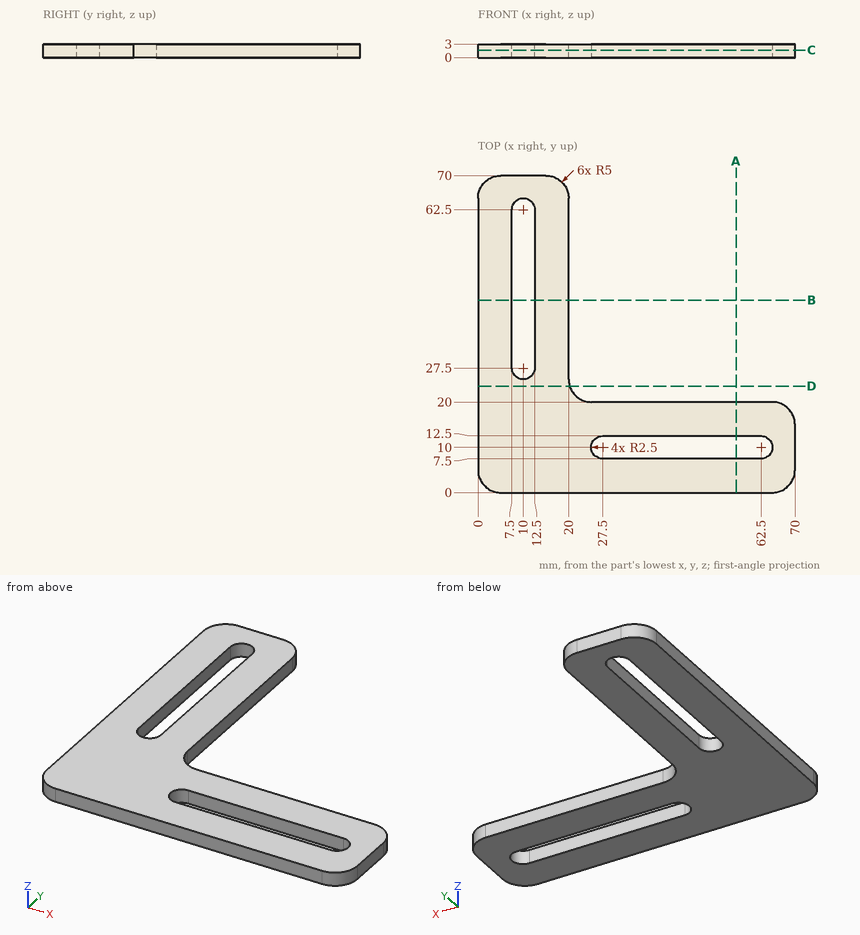
Source: three-view drawing plus pictorial views. Frame: mm from the lowest corner of the part. Coordinates: 2 decimals unless noted, no trailing zeros. Loops run counter-clockwise (first coordinate to the right, second up) from the corner with the lowest first, then second, coordinate; pieces in that order, holes last. Notation, with made-up numbers: (-39.5, 15.5) - (15.5, 15.5) arc R10 ccw to (15.5, 28.5) - close; hole circle Ø1 at (-34.5, 44). An arc over 180 degrees is marked (long way). Answer in a Markdown table with one row per item. Add a question column.
Item 1: Contact query for flat-ended pins moving along their axis: P1, Ø0.9, axis at y = 43.5, z = 2, coming from the +X side; P2, Ø1.5, axis at x = 49.5, z = 1, coming from the +Y side. Output: stop coordinate, or through.
Item 2: Section query A-A on x = 57. Return the cut outline in (y, z).
Item 3: Section query D-D on y = 23.5. Return the cut outline in (x, z).
Item 4: Section query C-C on z = 1.65. Return the cut outline in (x, y).
Item 5: Line query: line 1 along Y through (x, z) = (53, 2.4); line 2 along Y through (x, z) = (10, 1.1). Output: solid intervals per line, ascending. Write a range as [from, to].
Recorded:
| question | item | result |
|---|---|---|
| 1 | P1 | x = 20 |
| 1 | P2 | y = 20 |
| 2 | outline | (0, 0) - (7.5, 0) - (7.5, 3) - (0, 3) - close; (12.5, 0) - (20, 0) - (20, 3) - (12.5, 3) - close |
| 3 | outline | (0, 0) - (20.23, 0) - (20.23, 3) - (0, 3) - close |
| 4 | outline | (0, 5) arc R5 ccw to (5, 0) - (65, 0) arc R5 ccw to (70, 5) - (70, 15) arc R5 ccw to (65, 20) - (25, 20) arc R5 cw to (20, 25) - (20, 65) arc R5 ccw to (15, 70) - (5, 70) arc R5 ccw to (0, 65) - close; hole (7.5, 27.5) arc R2.5 ccw to (12.5, 27.5) - (12.5, 62.5) arc R2.5 ccw to (7.5, 62.5) - close; hole (27.5, 7.5) - (62.5, 7.5) arc R2.5 ccw to (62.5, 12.5) - (27.5, 12.5) arc R2.5 ccw to start |
| 5 | line 1 | [0, 7.5], [12.5, 20] |
| 5 | line 2 | [0, 25], [65, 70] |
